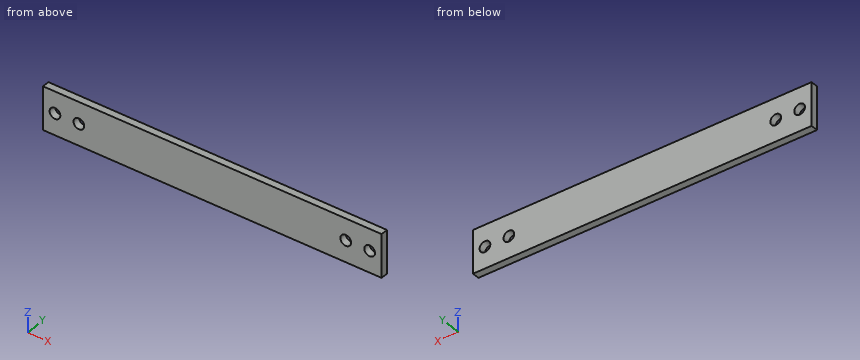
Autodesk Inventor part; units mm, degrees
ref_plane "YZ Plane" through (0, 0, 0) normal (1, 0, 0) x (0, 1, 0)
ref_plane "XZ Plane" through (0, 0, 0) normal (0, 1, 0) x (-1, 0, 0)
ref_plane "XY Plane" through (0, 0, 0) normal (0, 0, 1) x (1, 0, 0)
sketch "Sketch1" plane through (0, 0, 0) normal (0, 1, 0) x (-1, 0, 0)
  line L0 (-70.8, 9) -> (0, 9)
  line L1 (70.8, 9) -> (70.8, -9)
  line L2 (70.8, -9) -> (0, -9)
  line L3 (-70.8, -9) -> (-70.8, 9)
  line L4 (-70.8, 0) -> (70.8, 0) construction
  circle A0 centre (-65.8, 0) radius 2.25
  circle A1 centre (-55.8, 0) radius 2.25
  line L5 (0, 9) -> (70.8, 9)
  line L6 (0, -9) -> (-70.8, -9)
  line L7 (-50.8, 9) -> (-50.8, -9)
  line L8 (0, 37.7423) -> (0, -37.3462) construction
  circle A2 centre (65.8, 0) radius 2.25
  circle A3 centre (55.8, 0) radius 2.25
  line L9 (50.8, 9) -> (50.8, -9)
  point P0 (0, 0)
  dimension "d1" = 18
  dimension "d2" = 4.5
  dimension "d3" = 4.5
  dimension "d4" = 5
  dimension "d5" = 15
  dimension "d17" = 5
  dimension "d18" = 101.6
  dimension "d19" = 5
extrude "Extrusion1" add sketch "Sketch1" along normal blind 3
properties part number "TopSliderBar"
CAD build for the part. Positions are in the model's coordinates, mm. Round coordinates to 2 decimals unless told otherwise and drop trailing zeros. Write each loop counter-clockwise with the first axis right and the second up, starting at its lowest first coordinate (ties: lowest second). Pieces come first, ordered by that corner, then holes. Notation, with made-up numbers: (-7, 65) - (42, 65) arc R24 cw to (42, 84) - close; hole circle Ø1 at (61, 20.25). An arc over 180 degrees is marked (long way). Return JSON: item names as keys, results as strings. Group by question number.
Item 1: Band-saw the part on B-B on y = 1.8. List the corners of the cut face in (x, z).
Item 2: Probe probe 1 along X at (y, z) = (0.2, 0.25); probe 2 along Z at (x, y) = (-55.8, 1.25); probe 3 along Z at (x, y) = (-54.5, 1.9). List the from-to ranges inside material, lowest first.
Item 3: Band-saw the part on A-A on x = 55.8. List the corners of the cut face in (y, z).
Resolved:
{
 "1": {"outline": "(-70.8, -9) - (70.8, -9) - (70.8, 9) - (-70.8, 9) - close; hole circle Ø4.5 at (-65.8, 0); hole circle Ø4.5 at (-55.8, 0); hole circle Ø4.5 at (55.8, 0); hole circle Ø4.5 at (65.8, 0)"},
 "2": {"probe 1": "x = -70.8 to -68.04, -63.56 to -58.04, -53.56 to 53.56, 58.04 to 63.56, 68.04 to 70.8", "probe 2": "z = -9 to -2.25, 2.25 to 9", "probe 3": "z = -9 to -1.84, 1.84 to 9"},
 "3": {"outline": "(0, -9) - (3, -9) - (3, -2.25) - (0, -2.25) - close; (0, 2.25) - (3, 2.25) - (3, 9) - (0, 9) - close"}
}
